from build123d import *

# Parameters (mm, degrees)
SKETCH1_W           = 115
SKETCH1_H           = 100
SKETCH1_W_2         = 20
SKETCH1_H_2         = 3
BOSS_EXTRUDE1_DEPTH = 3
SKETCH2_R           = 6
CUT_EXTRUDE1_DEPTH  = 3
SKETCH3_R           = 2.6
CUT_EXTRUDE2_DEPTH  = 10


with BuildPart() as part:
    # Sketch1 → Boss-Extrude1 (new body)
    with BuildSketch(Plane.XY):
        with Locations((1, 0)):
            Rectangle(SKETCH1_W, SKETCH1_H)
        with Locations((-1.5, 51.5)):
            Rectangle(SKETCH1_W_2, SKETCH1_H_2)
        with Locations((-46.5, 51.5)):
            Rectangle(SKETCH1_W_2, SKETCH1_H_2)
    extrude(amount=BOSS_EXTRUDE1_DEPTH)

    # Sketch2 → Cut-Extrude1 (cut)
    with BuildSketch(Plane.XY.offset(3)):
        with Locations((-42.496090888, -34)):
            Circle(SKETCH2_R)
        with Locations((-42.496090888, -2)):
            Circle(SKETCH2_R)
        with Locations((-22.496090888, -34)):
            Circle(SKETCH2_R)
        with Locations((-22.496090888, -2)):
            Circle(SKETCH2_R)
    extrude(amount=-CUT_EXTRUDE1_DEPTH, mode=Mode.SUBTRACT)

    # Sketch3 → Cut-Extrude2 (cut)
    with BuildSketch(Plane.XY.offset(3)):
        with Locations((24.560133375, 20.17760104)):
            Circle(SKETCH3_R)
        with Locations((37.863702859, -12.19545935)):
            Circle(SKETCH3_R)
        with BuildLine():
            Line((1.884861427, -19.412788021), (20.117628398, -11.920111105))
            ThreePointArc((20.117628398, -11.920111105), (26.061223823, -11.099334991), (30.864513292, -7.503725129))
            Line((30.864513292, -7.503725129), (49.097066309, -0.010527574))
            ThreePointArc((49.097066309, -0.010527574), (50.035092062, 0.783146292), (50.33183638, 1.975519274))
            ThreePointArc((50.33183638, 1.975519274), (48.230377797, 10.984733419), (43.389811543, 18.868323086))
            ThreePointArc((43.389811543, 18.868323086), (42.334905798, 19.508804913), (41.104917855, 19.407944809))
            Line((41.104917855, 19.407944809), (22.86955388, 11.921590589))
            ThreePointArc((22.86955388, 11.921590589), (16.932809638, 11.096881192), (12.135486708, 7.503725129))
            Line((12.135486708, 7.503725129), (-6.097280263, 0.011048213))
            ThreePointArc((-6.097280263, 0.011048213), (-7.035570092, -0.78284909), (-7.33239795, -1.975557752))
            ThreePointArc((-7.33239795, -1.975557752), (-5.230898436, -10.984947373), (-0.3902379, -18.868690592))
            ThreePointArc((-0.3902379, -18.868690592), (0.659469027, -19.508046594), (1.884861427, -19.412788021))
        make_face()
        with Locations((18.439866625, -20.17760104)):
            Circle(SKETCH3_R)
        with Locations((5.136297141, 12.19545935)):
            Circle(SKETCH3_R)
    extrude(amount=-CUT_EXTRUDE2_DEPTH, mode=Mode.SUBTRACT)


solid = part.part
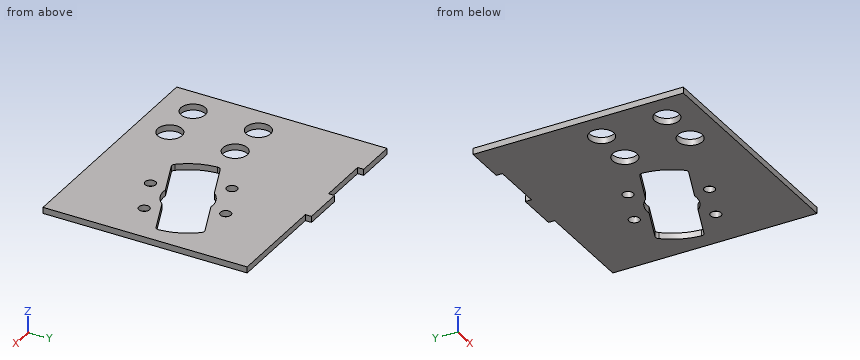
Work out the finished part from the listing and answer in its coordinate system (mm). Coordinates: 2 decimals unless noted, no trailing zeros. Order: outer loops, then holes, each group sorted by start corner. A loop starts at its lowest first (then second) coordinate and runs counter-clockwise, first axis right, second up. Notation, with made-up numbers: (47.25, 66) - (68.25, 66) arc R10 ccw to (68.25, 75) - close; hole circle Ø2 at (-6.5, 23.5). An arc over 180 degrees is marked (long way). Put each result on its own line as item: value. Start each with the question number.
1) Find section C-C (z = 2.45). State how many separate pieces and enclosed holes the cut face has, plus the area to 3 significant figures.
2) Find section B-B (y = -34). Give the vertices of the cut face in (x, z), plus the area to 3 significant figures.
3) Find the intervals of material crossed by line 1 (Y direction, x = -42.5, z = 0.35); line 2 (Y direction, x = 24.5, z = 0.45); line 3 (Y direction, x = -4.5, z = 2.3), in increasing order. Write a range as from..to.
4) Flat-ended cylindrical pins translate along their axes: pin 1 (3 mm diameter, centred on x = 5.14, y = 12.2, fed in from +Z); pin 2 (1.5 mm diameter, centred on x = 32.5, z = 1.5, fed in from +Y). Find the tip coordinate at first contact, or state that the pin passes through.
5) Find section A-A (x = -42.5). Give the vertices of the cut face in (y, z).
Results list:
1. separate pieces: 1
1. enclosed holes: 9
1. area: 9,870 mm^2
2. outline: (-56.5, 0) - (-48.5, 0) - (-48.5, 3) - (-56.5, 3) - close; (-36.5, 0) - (-28.5, 0) - (-28.5, 3) - (-36.5, 3) - close; (-16.5, 0) - (58.5, 0) - (58.5, 3) - (-16.5, 3) - close
2. area: 273 mm^2
3. line 1: y = -50..-40, -28..-8, 4..53
3. line 2: y = -50..-11.62, 12.59..17.58, 22.78..50
3. line 3: y = -50..-12.62, 0.67..53
4. pin 1: passes through
4. pin 2: stops at y = 50
5. outline: (-50, 0) - (-40, 0) - (-40, 3) - (-50, 3) - close; (-28, 0) - (-8, 0) - (-8, 3) - (-28, 3) - close; (4, 0) - (53, 0) - (53, 3) - (4, 3) - close
